The listing builds one solid part. Answer for the finished solid, in the listing's coordinates (mm). A direction names the side the tool comes from. Round coordinates to 2 decimals unless told otherwise and drop trailing zeros. Loops run counter-clockwise (first coordinate to the right, second up) from the corner with the lowest first, then second, coordinate; pieces in that order, holes last. Notation, with made-up numbers: (29, 29.25) -> (34, 29.25) arc R25 cw to (34, 57.25) -> close; hole circle Ø7 at (-18.75, 38). An arc over 180 degrees is marked (long way). Use a Markdown table: item, result. Add a question column.
Q1. For a pull along Z with two mould halves and no side action, classify faces 4 (the cylindrical face through (-2.53, 37.69, -43.96)), 5 (the flat face through (20, 10, -20)), 6 (the flat face through (-3, 49, 0)) as released by +Z, released by -Z, zero draft, split by the parting line, or undercut.
Q2. Section D-D on y = 40 is taken. Give the vertices of the cut face in (x, z).
Q3. Which of the six approach directions +Z, -Z, +X, -X, +Y, -Y give full straight-line access (tool end or side, diameter ignored) to faces 1 (the flat face through (3, 90, -16)), 2 (the flat face through (3, 70, -16)), 3 (the flat face through (7, 80, -30))?
Q4. Section A-A on y = 10 is taken. Give the vertices of the cut face in (x, z), then the cut area to 3 significant figures.
Q5. Section B-B on x = 1 is taken. Give the vertices of the cut face in (y, z).
Q6. Section C-C on z = -43 is taken. Give the vertices of the cut face in (x, y), then the cut area to 3 significant figures.
Q7. Given pin 1 Ø3 at (x, y) = (7.5, 80.5) entering from +Z; pin 2 Ø4.5 at (x, y) = (5, 14.5) entering from -Z; pin 3 Ø1 at (y, z) = (40.5, -13) entering from +X; pin 4 Ø3 at (y, z) = (40, -43) entering from -X (3 decimals), each flat-ended and moving along its own axis, determine where each tip first touches the part or whether it passes through.
Q8. Consider line 1 (Z direction, x = 9.5, y = 13); line 2 (Z direction, x = -1.35, y = 10); line 3 (X direction, y = 19, z = -3). Determine where each line is inside the solid, lowest interval first.
from build123d import *

# Parameters (mm, degrees)
F0_W     = 5
F0_H     = 50
F1_DEPTH = 100
F3_D     = 5
F2_W     = 20
F2_H     = 20
F4_DEPTH = 20
F5_SIZE  = 5
F7_D     = 15.5


with BuildPart() as f1:
    # F0 (on Front) → F1 (new body)
    with BuildSketch(Plane.XZ):
        with Locations((-2.5, -25)):
            Rectangle(F0_W, F0_H)
    extrude(amount=-F1_DEPTH)

    # F3 (through all)
    with Locations(Plane.YZ):
        with Locations((10, -43), (40, -43)):
            Hole(F3_D / 2)

    # F2 (on face) → F4 (join)
    with BuildSketch(Plane.YZ):
        with Locations((10, -20)):
            Rectangle(F2_W, F2_H)
        with Locations((80, -20)):
            Rectangle(F2_W, F2_H)
    extrude(amount=F4_DEPTH)

    # F5
    f5_edges = [f1.edges().sort_by_distance(p)[0] for p in [
        (20, 10, -10),
        (20, 10, -30),
        (20, 80, -10),
        (20, 80, -30),
    ]]
    chamfer(f5_edges, length=F5_SIZE)

    # F7 (through all)
    with Locations(Plane.XZ):
        with Locations((10, -20)):
            Hole(F7_D / 2)


solid = f1.part
Checked values:
| question | item | result |
|---|---|---|
| 1 | face 4 | undercut |
| 1 | face 5 | zero draft |
| 1 | face 6 | released by +Z |
| 2 | outline | (-5, -50) -> (0, -50) -> (0, -45.5) -> (-5, -45.5) -> close; (-5, -40.5) -> (0, -40.5) -> (0, 0) -> (-5, 0) -> close |
| 3 | face 1 | +Z, -Z, +X, +Y |
| 3 | face 2 | +Z, -Z, +X |
| 3 | face 3 | -Z, +X, +Y, -Y |
| 4 | outline | (-5, -50) -> (0, -50) -> (0, -45.5) -> (-5, -45.5) -> close; (-5, -40.5) -> (0, -40.5) -> (0, -30) -> (15, -30) -> (20, -25) -> (20, -15) -> (15, -10) -> (0, -10) -> (0, 0) -> (-5, 0) -> close; hole circle Ø15.5 at (10, -20) |
| 4 | area | 411 mm2 |
| 5 | outline | (0, -30) -> (20, -30) -> (20, -10) -> (0, -10) -> close; (70, -30) -> (90, -30) -> (90, -10) -> (70, -10) -> close |
| 6 | outline | (-5, 0) -> (0, 0) -> (0, 7.5) -> (-5, 7.5) -> close; (-5, 12.5) -> (0, 12.5) -> (0, 37.5) -> (-5, 37.5) -> close; (-5, 42.5) -> (0, 42.5) -> (0, 100) -> (-5, 100) -> close |
| 6 | area | 450 mm2 |
| 7 | pin 1 | stops at z = -10 |
| 7 | pin 2 | stops at z = -30 |
| 7 | pin 3 | stops at x = 0 |
| 7 | pin 4 | passes through |
| 8 | line 1 | z = -30 to -27.73, -12.27 to -10 |
| 8 | line 2 | z = -50 to -45.5, -40.5 to 0 |
| 8 | line 3 | x = -5 to 0 |
